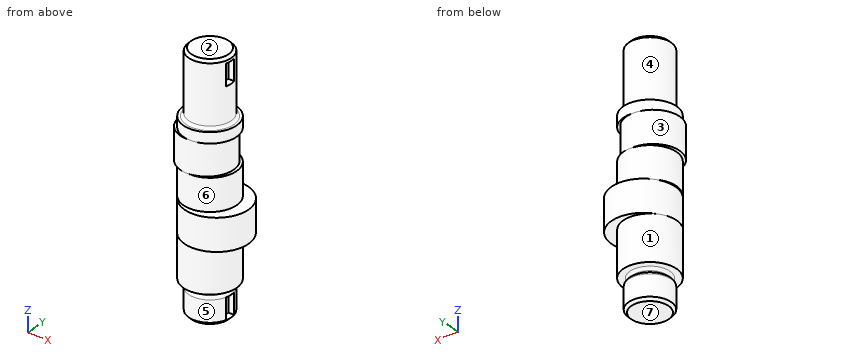
from build123d import *

# Parameters (mm, degrees)
SKETCH_1_R          = 8
EXTRUDE_1_DEPTH     = 10
SKETCH_2_R          = 6.5
EXTRUDE_2_DEPTH     = 2
SKETCH_3_R          = 10
EXTRUDE_3_DEPTH     = 17
SKETCH_4_R          = 12
EXTRUDE_4_DEPTH     = 12
SKETCH_5_R          = 10
EXTRUDE_5_DEPTH     = 12
SKETCH_6_R          = 10
EXTRUDE_6_DEPTH     = 12
SKETCH_7_R          = 10
EXTRUDE_7_DEPTH     = 4
SKETCH_8_R          = 8
EXTRUDE_8_DEPTH     = 24
SKETCH_9_W          = 5.5
SKETCH_9_H          = 4
CUT_EXTRUDE_1_DEPTH = 8
SKETCH_10_W         = 5.5
SKETCH_10_H         = 4
CUT_EXTRUDE_2_DEPTH = 8
CHAMFER_1_SIZE      = 1
FILLET_1_R          = 1


with BuildPart() as part:
    # 草图1 → 凸台-拉伸1 (new body)
    with BuildSketch(Plane.XY.offset(-13)):
        Circle(SKETCH_1_R)
    extrude(amount=EXTRUDE_1_DEPTH)

    # 草图2 → 凸台-拉伸2 (add)
    with BuildSketch(Plane.XY.offset(-3)):
        Circle(SKETCH_2_R)
    extrude(amount=EXTRUDE_2_DEPTH)

    # 草图3 → 凸台-拉伸3 (add)
    with BuildSketch(Plane.XY.offset(-1)):
        Circle(SKETCH_3_R)
    extrude(amount=EXTRUDE_3_DEPTH)

    # 草图4 → 凸台-拉伸4 (add)
    with BuildSketch(Plane.XY.offset(16)):
        with Locations(Location((2.5, 0, 0), (0, 0, 213.122940208))):
            Circle(SKETCH_4_R)
    extrude(amount=EXTRUDE_4_DEPTH)

    # 草图5 → 凸台-拉伸5 (add)
    with BuildSketch(Plane.XY.offset(28)):
        with Locations(Location((0, 0, 0), (0, 0, 139.025369771))):
            Circle(SKETCH_5_R)
    extrude(amount=EXTRUDE_5_DEPTH)

    # 草图6 → 凸台-拉伸6 (add)
    with BuildSketch(Plane.XY.offset(40)):
        with Locations(Location((-1.2, 0, 0), (0, 0, 273.439812768))):
            Circle(SKETCH_6_R)
    extrude(amount=EXTRUDE_6_DEPTH)

    # 草图7 → 凸台-拉伸7 (add)
    with BuildSketch(Plane.XY.offset(52)):
        with Locations(Location((0, 0, 0), (0, 0, 139.025369771))):
            Circle(SKETCH_7_R)
    extrude(amount=EXTRUDE_7_DEPTH)

    # 草图8 → 凸台-拉伸8 (add)
    with BuildSketch(Plane.XY.offset(56)):
        Circle(SKETCH_8_R)
    extrude(amount=EXTRUDE_8_DEPTH)

    # 草图9 → 切除-拉伸1 (cut)
    with BuildSketch(Plane.XY.offset(-12)):
        with Locations((8.25, 0)):
            Rectangle(SKETCH_9_W, SKETCH_9_H)
    extrude(amount=CUT_EXTRUDE_1_DEPTH, mode=Mode.SUBTRACT)

    # 草图10 → 切除-拉伸2 (cut)
    with BuildSketch(Plane.XY.offset(70)):
        with Locations((8.25, 0)):
            Rectangle(SKETCH_10_W, SKETCH_10_H)
    extrude(amount=CUT_EXTRUDE_2_DEPTH, mode=Mode.SUBTRACT)

    # 倒角1
    chamfer_1_edges = [part.edges().sort_by_distance(p)[0] for p in [
        (-8, 0, -13),
        (-8, 0, 80),
    ]]
    chamfer(chamfer_1_edges, length=CHAMFER_1_SIZE - 0.0001)  # a hair under: the kernel refuses the full size

    # 圆角1
    fillet_1_edges = [part.edges().sort_by_distance(p)[0] for p in [
        (-8, 0, 56),
        (-8, 0, -3),
        (-6.5, 0, -1),
    ]]
    fillet(fillet_1_edges, radius=FILLET_1_R - 0.0001)  # a hair under: the kernel refuses the full size


solid = part.part
The model under review builds one solid part; all positions refer to its coordinate system, in mm. Face numbers are marked on the shaded views. A direction names the side the tool comes from. Coordinates: 2 decimals unless noted, no trailing zeros. Write each loop counter-clockwise with the first axis right and the second up, starting at its lowest first coordinate (ties: lowest second). Pieces come first, ordered by that corner, then holes. Notation, with made-up numbers: (-2, -25.5) - (53, -25.5) arc R25 cw to (53, -5.5) - close; hole circle Ø5 at (29, -9). An arc over 180 degrees is marked (long way). Answer as CSV lines item,"result".
(1) Clearance check with flat-ended pins moving along their axes: pin 1 Ø10 at (x, z) = (8.5, 38) entering from +Y; pin 2 Ø2.5 at (x, y) = (-9, -1) entering from +Z; pin 3 Ø1.1 at (x, z) = (6.5, 72.5) entering from -Y. State where each tip first meets the part, or that it passes through.
Data:
pin 1,"stops at y = 9.37"
pin 2,"stops at z = 79.19"
pin 3,"stops at y = -5.35"
(2) Tool access review of the marked faces 1, 2, 3 and 4: name each direction out of +Z, -Z, +X, -X, +Y, -Y from which nothing blocks a thin tool from reaching the whole face with its end or side.
Data:
face 1,"-Z"
face 2,"+Z, +X, -X, +Y, -Y"
face 3,"none"
face 4,"+Z"
(3) Mouldability with a two-part tool opening along Z and no side actions: class the marked faces 5, 6 and 7 as pulls with the +Z half, pulls with the -Z half, needs draft (parallel to the pull), parting line crosses it, or undercut.
Data:
face 5,"needs draft"
face 6,"undercut"
face 7,"pulls with the -Z half"
(4) We need section A-A (z = -5). Give the boundary of the cut face in (x, y).
Data:
outline,"(5.5, -2) - (5.5, 2) - (7.75, 2) arc R8 ccw (long way) to (7.75, -2) - close"
(5) We need section B-B (x = 12.25). Give the boundary of the cut face in (y, z), plus the area to 3 significant figures.
Data:
outline,"(-7, 16) - (7, 16) - (7, 28) - (-7, 28) - close"
area,"168 mm2"
(6) We need section C-C (z = 39). Give the boundary of the cut face in (x, y), plus the area to 3 significant figures.
Data:
outline,"circle Ø20 at (0, 0)"
area,"314 mm2"
(7) For line 1 along Z through (x, y) = (5.75, -0.25); line 2 along Y through (x, z) = (-1.75, 43.5); line 3 along Z through (x, y) = (3.25, -8.5), list the stretches that pass through material, from the lowest coordinate up. Write a range as [from, to].
Data:
line 1,"z = [-13, -12], [-4, 70], [78, 80]"
line 2,"y = [-9.98, 9.98]"
line 3,"z = [-1, 56]"
